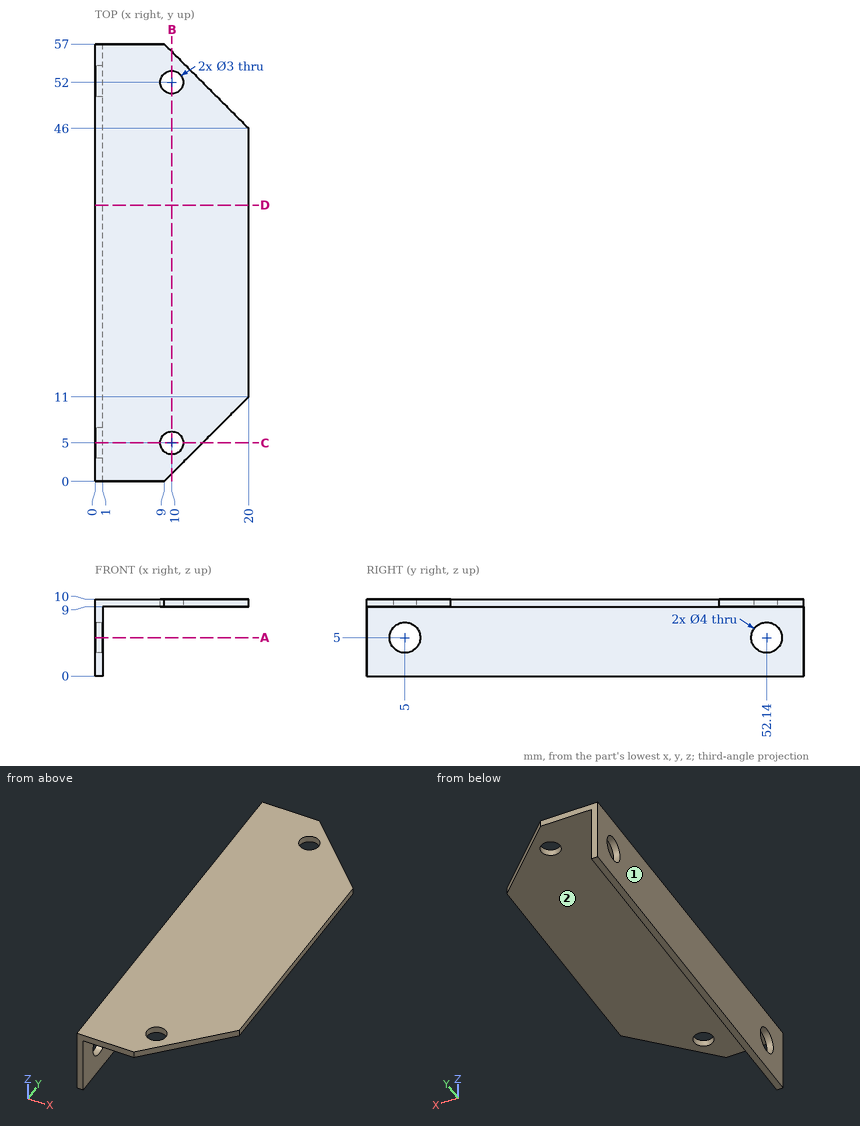
Study the drawing (mm; zero at the part's minimum x, y, z) and answer. A direction names the side the tool comes from. Round coordinates to 2 decimals unless told otherwise and drop trailing zeros. Write each loop counter-clockwise with the first axis right and the second up, starting at its lowest first coordinate (ties: lowest second). Pieces come first, ordered by that corner, then holes. Notation, with made-up numbers: (8.5, 34) -> (21.5, 34) arc R15 ccw to (21.5, 44) -> close; hole circle Ø9 at (-5.5, 77). An arc over 180 degrees is marked (long way). Answer as CSV lines item,"result". Start each with the question number.
(1) Each of these flat-tipped pins is pushed along its axis until it touches: pin 1 (1.5 mm diameter, centred on y = 28.5, z = 6, fed in from -X); pin 2 (5.5 mm diameter, centred on x = 10, y = 23, fed in from -Z); pin 3 (5 mm diameter, centred on x = 15, z = 7, fed in from +Y); pin 4 (3.5 mm diameter, centred on y = 52.14, z = 5, fed in from -X). Where does it stop, or does it pass through?
(2) The part is cut by section B-B, the plane x = 10. Give the vertices of the cut face in (y, z).
(3) The part is cut by section C-C, the plane y = 5. Give the vertices of the cut face in (x, z), then the cut area to 3 significant figures.
(4) A tool of negligible diameter and unlimited length cuts with its end or side. For the marked faces 1 and 2, from which of +Z, -Z, +X, -X, +Y, -Y can it reach the whole face along a straight path? Write none if from no direction.
(5) Find the intervals of material crossed by probe 1 along Y at (x, z) = (0.3, 5); probe 2 along Z at (x, y) = (18, 11); probe 3 along X at (y, z) = (16.5, 2.75), in increasing order.
(6) The part is cut by section A-A, the plane z = 5. Give the vertices of the cut face in (x, y), then the cut area to 3 significant figures.
(7) The part is cut by section D-D, the plane y = 36. Give the vertices of the cut face in (x, z).
Output values:
1,pin 1,"stops at x = 0"
1,pin 2,"stops at z = 9"
1,pin 3,"stops at y = 52.5"
1,pin 4,"passes through"
2,outline,"(1, 9) -> (3.5, 9) -> (3.5, 10) -> (1, 10) -> close; (6.5, 9) -> (50.5, 9) -> (50.5, 10) -> (6.5, 10) -> close; (53.5, 9) -> (56, 9) -> (56, 10) -> (53.5, 10) -> close"
3,outline,"(0, 0) -> (1, 0) -> (1, 3) -> (0, 3) -> close; (0, 7) -> (1, 7) -> (1, 9) -> (8.5, 9) -> (8.5, 10) -> (0, 10) -> close; (11.5, 9) -> (14, 9) -> (14, 10) -> (11.5, 10) -> close"
3,area,"16.0 mm²"
4,face 1,"+Z, -Z, -X, +Y, -Y"
4,face 2,"-Z, +X, +Y, -Y"
5,probe 1,"y = 0 to 3, 7 to 50.14, 54.14 to 57"
5,probe 2,"z = 9 to 10"
5,probe 3,"x = 0 to 1"
6,outline,"(0, 0) -> (1, 0) -> (1, 3) -> (0, 3) -> close; (0, 7) -> (1, 7) -> (1, 50.14) -> (0, 50.14) -> close; (0, 54.14) -> (1, 54.14) -> (1, 57) -> (0, 57) -> close"
6,area,"49.0 mm²"
7,outline,"(0, 0) -> (1, 0) -> (1, 9) -> (20, 9) -> (20, 10) -> (0, 10) -> close"
